from build123d import *

# Parameters (mm, degrees)
F0_R     = 11.1
F1_DEPTH = 7


with BuildPart() as f1:
    # F0 (on Front) → F1 (new body)
    with BuildSketch(Plane.XZ):
        with BuildLine():
            ThreePointArc((6.2338166768, 15.8158), (0, 13.9), (-6.2338166768, 15.8158))
            ThreePointArc((-6.2338166768, 15.8158), (-6.9759049464, 15.5027981403), (-7.7023356847, 15.155))
            ThreePointArc((-7.7023356847, 15.155), (-11.1819106583, 6.4554763423), (-16.9757337999, -0.9079988747))
            ThreePointArc((-16.9757337999, -0.9079988747), (-16.9137232859, -1.71054512), (-16.8137929196, -2.5092563954))
            ThreePointArc((-16.8137929196, -2.5092563954), (-12.2458770397, -6.6041942087), (-10.5506350946, -12.5))
            ThreePointArc((-10.5506350946, -12.5), (-10.557972807, -12.9035385636), (-10.5799762428, -13.3065436046))
            ThreePointArc((-10.5799762428, -13.3065436046), (-9.9377854009, -13.7927669931), (-9.2732836372, -14.2480247959))
            ThreePointArc((-9.2732836372, -14.2480247959), (0.0003631141, -12.0362492821), (9.2741432999, -14.2474652501))
            ThreePointArc((9.2741432999, -14.2474652501), (9.9382015017, -13.79246718), (10.5799762428, -13.3065436046))
            ThreePointArc((10.5799762428, -13.3065436046), (12.0377531126, -6.95), (16.8137929196, -2.5092563954))
            ThreePointArc((16.8137929196, -2.5092563954), (16.9137310645, -1.7104682038), (16.9757420575, -0.9078444785))
            ThreePointArc((16.9757420575, -0.9078444785), (16.9939344323, -0.4540842556), (17, 0))
            ThreePointArc((17, 0), (10.6273382236, 6.5199223601), (7.7023356847, 15.155))
            ThreePointArc((7.7023356847, 15.155), (6.9759049464, 15.5027981403), (6.2338166768, 15.8158))
        make_face()
        Circle(F0_R, mode=Mode.SUBTRACT)
        with BuildLine():
            ThreePointArc((6.2338166768, 15.8158), (9.8082966185, 19.8031435036), (11.1, 25))
            ThreePointArc((11.1, 25), (-5.1968564964, 34.8082966185), (-6.2338166768, 15.8158))
            ThreePointArc((-6.2338166768, 15.8158), (0, 13.9), (6.2338166768, 15.8158))
        make_face()
        with BuildLine():
            ThreePointArc((-6.2338166768, 15.8158), (-5.1968564964, 34.8082966185), (11.1, 25))
            ThreePointArc((11.1, 25), (9.8082966185, 19.8031435036), (6.2338166768, 15.8158))
            ThreePointArc((6.2338166768, 15.8158), (6.9759049464, 15.5027981403), (7.7023356847, 15.155))
            ThreePointArc((7.7023356847, 15.155), (0, 37.5), (-7.7023356847, 15.155))
            ThreePointArc((-7.7023356847, 15.155), (-6.9759049464, 15.5027981403), (-6.2338166768, 15.8158))
        make_face()
        with BuildLine():
            ThreePointArc((-16.8137929196, -2.5092563954), (-16.9137232859, -1.71054512), (-16.9757337999, -0.9079988747))
            ThreePointArc((-16.9757337999, -0.9079988747), (-32.4756988834, -18.751271821), (-9.2732836372, -14.2480247959))
            ThreePointArc((-9.2732836372, -14.2480247959), (-9.9377854009, -13.7927669931), (-10.5799762428, -13.3065436046))
            ThreePointArc((-10.5799762428, -13.3065436046), (-31.2635170766, -18.05), (-16.8137929196, -2.5092563954))
        make_face()
        with BuildLine():
            ThreePointArc((9.2741432999, -14.2474652501), (32.4767837776, -18.7503949231), (16.9757420575, -0.9078444785))
            ThreePointArc((16.9757420575, -0.9078444785), (16.9137310645, -1.7104682038), (16.8137929196, -2.5092563954))
            ThreePointArc((16.8137929196, -2.5092563954), (27.5464408859, -3.0952419451), (32.7506350946, -12.5))
            ThreePointArc((32.7506350946, -12.5), (22.0541736582, -23.5926622876), (10.5799762428, -13.3065436046))
            ThreePointArc((10.5799762428, -13.3065436046), (9.9382015017, -13.79246718), (9.2741432999, -14.2474652501))
        make_face()
        with BuildLine():
            ThreePointArc((-10.5506350946, -12.5), (-12.2458770397, -6.6041942087), (-16.8137929196, -2.5092563954))
            ThreePointArc((-16.8137929196, -2.5092563954), (-31.2635170766, -18.05), (-10.5799762428, -13.3065436046))
            ThreePointArc((-10.5799762428, -13.3065436046), (-10.557972807, -12.9035385636), (-10.5506350946, -12.5))
        make_face()
        with BuildLine():
            ThreePointArc((32.7506350946, -12.5), (27.5464408859, -3.0952419451), (16.8137929196, -2.5092563954))
            ThreePointArc((16.8137929196, -2.5092563954), (12.0377531126, -6.95), (10.5799762428, -13.3065436046))
            ThreePointArc((10.5799762428, -13.3065436046), (22.0541736582, -23.5926622876), (32.7506350946, -12.5))
        make_face()
    extrude(amount=F1_DEPTH)


solid = f1.part
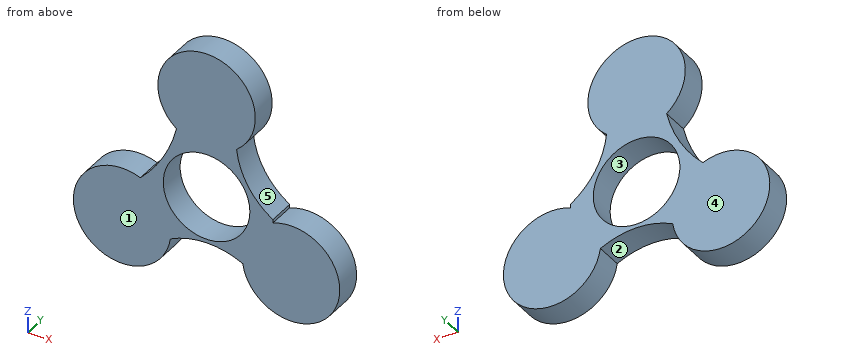
For this review, take the finished solid that the model builds, in its own axes (mm). Face numbers are marked on the shaded views. A direction names the side the tool comes from. Round coordinates to 2 decimals unless told otherwise and drop trailing zeros. Order: outer loops, then holes, each group sorted by start corner. A loop starts at its lowest first (then second) coordinate and runs counter-clockwise, first axis right, second up. Notation, with made-up numbers: M 12.25,36 L 27.25,36 A11 ccw 27.25,51 Z; hole C 76,70.25 d11. An arc over 180 degrees is marked long. Write each question's results on one line, items separated by ' | '. Start each with the question number.
1. Add section D-D (z = 25). State the section outline as (x, y) points.
2. Clearance check with flat-ended pins moving along their axes: pin 1 Ø1.5 at (y, z) = (-5.5, 8.5) entering from +X; pin 2 Ø4 at (y, z) = (-4, 6.5) entering from -X; pin 3 Ø1 at (x, y) = (15.5, -4) entering from -Z. State where each tip first meets the part, or that it passes through.
3. To check wall thickness, follow L1, parallel to Z at x = 0, y = -1.25; L2, parallel to Z at x = -4, y = -5.25; L3, parallel to X at y = -4.25, z = 1. State the ranges of each line that lie inside material, in increasing order. Write a range as [from, to].
4. Add section B-B (z = 7.5). State the section outline as (x, y) points.
5. Add section A-A (x = 0). State the section outline as (y, z) points, then the cut area to 3 significant figures.
6. Tool access review of the marked faces 4 and 5: name each direction out of +Z, -Z, +X, -X, +Y, -Y from which nothing blocks a thin tool from reaching the whole face with its end or side.
7. Draft analysis for pull direction Z (two halves, no side actions). For the marked faces 1, 2 and 3, state which applies: pulls with the +Z half, pulls with the -Z half, needs draft (parallel to the pull), parting line crosses it, or undercut.
Output values:
1) outline: M -12.5,-7 L 12.5,-7 L 12.5,0 L -12.5,0 Z
2) pin 1: x = 9.93 | pin 2: x = -12.4 | pin 3: z = -23.65
3) L1: [-12.04, -11.1], [11.1, 37.5] | L2: [-12.43, -10.35], [10.35, 36.84] | L3: [-15.13, -11.05], [11.05, 15.59]
4) outline: M -10.6,-7 L -8.18,-7 L -8.18,0 L -10.6,0 Z; M 8.18,-7 L 10.06,-7 L 10.06,0 L 8.18,0 Z
5) outline: M -7,-12.04 L 0,-12.04 L 0,-11.1 L -7,-11.1 Z; M -7,11.1 L 0,11.1 L 0,37.5 L -7,37.5 Z | area: 191 mm^2
6) face 4: +Z, -Z, +X, -X, +Y | face 5: +X, +Y, -Y
7) face 1: needs draft | face 2: pulls with the -Z half | face 3: undercut
